Source: CAD feature listing. Evaluate the final solid. Frame: model axes, mm. A direction names the side the tool comes from. Give positions to 0.01 mm unless a question says otherwise; leave off trailing zeros. Order: outer loops, then holes, each group sorted by start corner. A loop starts at its lowest first (then second) coordinate and runs counter-clockwise, first axis right, second up. Notation, with made-up numbers: (36, -2.75) - (71, -2.75) arc R17 cw to (71, 15.25) - close; hole circle Ø10 at (41.5, 53.5). An arc over 180 degrees is marked (long way). Answer as CSV lines item,"result".
```python
from build123d import *

# Parameters (mm, degrees)
SKETCH_W      = 203.2
SKETCH_H      = 44.45
SKETCH_R      = 2.775
SKETCH_W_2    = 98
SKETCH_H_2    = 19.1
PAD_DEPTH     = 2.2
SKETCH001_W   = 102
SKETCH001_H   = 23.1
SKETCH001_W_2 = 98
SKETCH001_H_2 = 19.1
PAD001_DEPTH  = 95.8
SKETCH002_W   = 102
SKETCH002_H   = 23.1
SKETCH002_W_2 = 88
SKETCH002_H_2 = 19.1
PAD002_DEPTH  = 2.2


with BuildPart() as part:
    # Sketch → Pad (new body)
    with BuildSketch(Plane.XY):
        Rectangle(SKETCH_W, SKETCH_H)
        with Locations((-93.6625, 15.875)):
            Circle(SKETCH_R, mode=Mode.SUBTRACT)
        with Locations((-93.6625, -15.875)):
            Circle(SKETCH_R, mode=Mode.SUBTRACT)
        with Locations((93.6625, 15.875)):
            Circle(SKETCH_R, mode=Mode.SUBTRACT)
        with Locations((93.6625, -15.875)):
            Circle(SKETCH_R, mode=Mode.SUBTRACT)
        Rectangle(SKETCH_W_2, SKETCH_H_2, mode=Mode.SUBTRACT)
    extrude(amount=PAD_DEPTH)

    # Sketch001 (on Face14 of Pad) → Pad001 (join)
    with BuildSketch(Plane.XY.offset(2.2)):
        Rectangle(SKETCH001_W, SKETCH001_H)
        Rectangle(SKETCH001_W_2, SKETCH001_H_2, mode=Mode.SUBTRACT)
    extrude(amount=PAD001_DEPTH)

    # Sketch002 (on Face23 of Pad001) → Pad002 (join)
    with BuildSketch(Plane.XY.offset(98)):
        Rectangle(SKETCH002_W, SKETCH002_H)
        Rectangle(SKETCH002_W_2, SKETCH002_H_2, mode=Mode.SUBTRACT)
    extrude(amount=PAD002_DEPTH)


solid = part.part
```
(1) Access query for faces 4 (the flat face through (-49, 0, 48)), 5 (the cylindrical face through (-91.1, 14.81, 1.08)), 6 (the flat face through (51, 0, 51)), 7 (the flat face through (-1, 11.55, 51)), 8 (the flat face through (-1, -11.55, 51)). Directions: +Z, -Z, +X, -X, +Y, -Y. A direction counts if a zero-diameter tool reaches every point of the face in a straight line with its end or side. Return the directions, or none.
Completed:
face 4,"-Z"
face 5,"+Z, -Z"
face 6,"+Z, +X, +Y, -Y"
face 7,"+Z, +X, -X, +Y"
face 8,"+Z, +X, -X, -Y"
(2) Cut plane C-C (y = 7). Return loops of the section in (x, z), then the cut area to 3 significant figures.
Completed:
outline,"(-101.6, 0) - (-49, 0) - (-49, 98) - (-44, 98) - (-44, 100.2) - (-51, 100.2) - (-51, 2.2) - (-101.6, 2.2) - close; (44, 98) - (49, 98) - (49, 0) - (101.6, 0) - (101.6, 2.2) - (51, 2.2) - (51, 100.2) - (44, 100.2) - close"
area,"645 mm²"
(3) Cut plane B-B (x = -46). Return loops of the section in (y, z) (3 decimals), then the cut area to 3 significant figures.
Completed:
outline,"(-22.225, 0) - (-9.55, 0) - (-9.55, 98) - (9.55, 98) - (9.55, 0) - (22.225, 0) - (22.225, 2.2) - (11.55, 2.2) - (11.55, 100.2) - (-11.55, 100.2) - (-11.55, 2.2) - (-22.225, 2.2) - close"
area,"490 mm²"
(4) Cut plane A-A (z = 36). Return loops of the section in (x, y).
Completed:
outline,"(-51, -11.55) - (51, -11.55) - (51, 11.55) - (-51, 11.55) - close; hole (-49, -9.55) - (49, -9.55) - (49, 9.55) - (-49, 9.55) - close"
(5) Cut plane D-D (x = 32). Return loops of the section in (y, z) (3 decimals), then the cut area to 3 significant figures.
Completed:
outline,"(-22.225, 0) - (-9.55, 0) - (-9.55, 100.2) - (-11.55, 100.2) - (-11.55, 2.2) - (-22.225, 2.2) - close; (9.55, 0) - (22.225, 0) - (22.225, 2.2) - (11.55, 2.2) - (11.55, 100.2) - (9.55, 100.2) - close"
area,"448 mm²"
(6) Ray query, line 1 (Y direction, x = 1.5, z = 44); line 2 (X direction, y = -9.5, z = 32.5); line 3 (Z direction, x = 80, y = -2.5). Return the intervals inside material, ascending. Write a range as from..to.
Completed:
line 1,"-11.55..-9.55, 9.55..11.55"
line 2,"-51..-49, 49..51"
line 3,"0..2.2"
(7) Mould query, pull axis X, two halves, no side actions, for faces 1 (the flat face through (-1, -10, 100.2)), 2 (the flat face through (-1, -9.55, 49)), 3 (the flat face through (-51, 0, 51)). Classes: released by +X, released by -X, zero draft, split by the parting line, or undercut.
Completed:
face 1,"zero draft"
face 2,"undercut"
face 3,"released by -X"
(8) Contact query for flat-ended pins moving along their axis: pin 1 (4 mm diameter, centred on x = -46, y = -4.5, fed in from -Z); pin 2 (3 mm diameter, centred on y = -11.5, z = 13.5, fed in from -X); pin 3 (5 mm diameter, centred on x = 72, y = 3, fed in from +Z); pin 4 (8 mm diameter, centred on y = -17, z = 83, fed in from -X). Output: stop coordinate, or through.
Completed:
pin 1,"z = 98"
pin 2,"x = -51"
pin 3,"z = 2.2"
pin 4,"through"
